Geometry check sheet. Reference: the model listing, model coordinates, mm. A direction names the side the tool comes from. Coordinates: 2 decimals unless noted, no trailing zeros. Loops run counter-clockwise (first coordinate to the right, second up) from the corner with the lowest first, then second, coordinate; pieces in that order, holes last.
from build123d import *

# Parameters (mm, degrees)
SKETCH1_W               = 58
SKETCH1_H               = 48
SKETCH1_R               = 13
SKETCH1_R_2             = 1.8
BOSS_EXTRUDE1_DEPTH     = 5
BOSS_EXTRUDE2_OUTLINE_R = 4.2
BOSS_EXTRUDE2_DEPTH     = 10
FILLET1_R               = 5
BOSS_EXTRUDE5_DEPTH     = 10
CUT_EXTRUDE2_DEPTH      = 67.492480778
SKETCH7_W               = 58
SKETCH7_H               = 5
BOSS_EXTRUDE6_DEPTH     = 13
SKETCH8_R               = 3.3
SKETCH8_R_2             = 1.8
CUT_EXTRUDE3_DEPTH      = 20


# Read off the part's stored shape, not the designer's step: Boss-Extrude2, Boss-Extrude5
with BuildPart() as part:
    # Sketch1 → Boss-Extrude1 (new body)
    with BuildSketch(Plane(origin=(0, 0, 0), x_dir=(1, 0, 0), z_dir=(0, 1, 0))):
        with Locations((29, -24)):
            Rectangle(SKETCH1_W, SKETCH1_H)
        with Locations(Location((35.15, -26.15, 0), (0, 0, 270))):
            Circle(SKETCH1_R, mode=Mode.SUBTRACT)
        with Locations(Location((19.65, -10.65, 0), (0, 0, 270))):
            Circle(SKETCH1_R_2, mode=Mode.SUBTRACT)
        with Locations(Location((19.65, -41.65, 0), (0, 0, 270))):
            Circle(SKETCH1_R_2, mode=Mode.SUBTRACT)
        with Locations(Location((50.65, -41.65, 0), (0, 0, 270))):
            Circle(SKETCH1_R_2, mode=Mode.SUBTRACT)
        with Locations(Location((50.65, -10.65, 0), (0, 0, 270))):
            Circle(SKETCH1_R_2, mode=Mode.SUBTRACT)
    extrude(amount=BOSS_EXTRUDE1_DEPTH)

    # Boss-Extrude2 outline → Boss-Extrude2 (add)
    with BuildSketch(Plane(origin=(0, 5, 0), x_dir=(1, 0, 0), z_dir=(0, 1, 0))):
        with BuildLine():
            ThreePointArc((23.271694215, -31.432598951), (22.15, -26.15), (23.271694215, -20.867401049))
            ThreePointArc((23.271694215, -20.867401049), (8.8, -26.15), (23.271694215, -31.432598951))
        make_face()
        with Locations((17, -26.15)):
            Circle(BOSS_EXTRUDE2_OUTLINE_R, mode=Mode.SUBTRACT)
    extrude(amount=BOSS_EXTRUDE2_DEPTH)

    # Fillet1
    fillet1_edges = [part.edges().sort_by_distance(p)[0] for p in [
        (58, 2.5, 48),
        (0, 2.5, 48),
    ]]
    fillet(fillet1_edges, radius=FILLET1_R)

    # Boss-Extrude5 outline → Boss-Extrude5 (add)
    with BuildSketch(Plane(origin=(0, 5, 0), x_dir=(1, 0, 0), z_dir=(0, 1, 0))):
        with BuildLine():
            ThreePointArc((19.5, -12.443739111), (17.85, -10.65), (19.5, -8.856260889))
            Line((19.5, -8.856260889), (19.5, -5))
            Line((19.5, -5), (14.5, -5))
            Line((14.5, -5), (14.5, -18.340390535))
            ThreePointArc((14.5, -18.340390535), (17, -17.95), (19.5, -18.340390535))
            Line((19.5, -18.340390535), (19.5, -12.443739111))
        make_face()
        with BuildLine():
            ThreePointArc((19.5, -33.959609465), (17, -34.35), (14.5, -33.959609465))
            Line((14.5, -33.959609465), (14.5, -48))
            Line((14.5, -48), (19.5, -48))
            Line((19.5, -48), (19.5, -43.443739111))
            ThreePointArc((19.5, -43.443739111), (17.85, -41.65), (19.5, -39.856260889))
            Line((19.5, -39.856260889), (19.5, -33.959609465))
        make_face()
    extrude(amount=BOSS_EXTRUDE5_DEPTH)

    # Sketch6 → Cut-Extrude2 (cut, through all)
    with BuildSketch(Plane.ZY.offset(-14.5)):
        Polygon((17.340390535, 15), (5, 6), (5, 15), align=None)
        Polygon((48, 6), (34.959609465, 15), (48, 15), align=None)
    extrude(amount=-CUT_EXTRUDE2_DEPTH, mode=Mode.SUBTRACT)

    # Sketch7 → Boss-Extrude6 (add)
    with BuildSketch(Plane(origin=(0, 5, 0), x_dir=(1, 0, 0), z_dir=(0, 1, 0))):
        with Locations((29, -2.5)):
            Rectangle(SKETCH7_W, SKETCH7_H)
    extrude(amount=BOSS_EXTRUDE6_DEPTH)

    # Sketch8 → Cut-Extrude3 (cut)
    with BuildSketch(Plane.XY.offset(5)):
        with Locations((35, 11.5)):
            Circle(SKETCH8_R)
        with Locations((50, 11.5)):
            Circle(SKETCH8_R_2)
    extrude(amount=-CUT_EXTRUDE3_DEPTH, mode=Mode.SUBTRACT)


solid = part.part
(1) Scan lines: L1, parallel to X at y = 2.05, z = 41.65; L2, parallel to Z at x = 35.15, y = 3.8; L3, parallel to Z at x = 19.65, y = 2.1. Record each from-to range of solid material in increasing order.
Findings:
L1: x = 0 to 17.85, 21.45 to 48.85, 52.45 to 58
L2: z = 0 to 13.15, 39.15 to 48
L3: z = 0 to 8.85, 12.45 to 39.85, 43.45 to 48
(2) Sectioned sample at D-D on z = 41. Record the cut outline in (x, y).
Findings:
outline: (0, 0) - (17.97, 0) - (17.97, 10.83) - (14.5, 10.83) - (14.5, 5) - (0, 5) - close; (21.33, 0) - (48.97, 0) - (48.97, 5) - (21.33, 5) - close; (52.33, 0) - (58, 0) - (58, 5) - (52.33, 5) - close
(3) Sectioned sample at A-A on y = 1.75. Record the cut outline in (x, z).
Findings:
outline: (0, 0) - (58, 0) - (58, 43) arc R5 ccw to (53, 48) - (5, 48) arc R5 ccw to (0, 43) - close; hole circle Ø3.6 at (19.65, 10.65); hole circle Ø3.6 at (19.65, 41.65); hole circle Ø26 at (35.15, 26.15); hole circle Ø3.6 at (50.65, 10.65); hole circle Ø3.6 at (50.65, 41.65)
(4) Sectioned sample at B-B on x = 50.65. Record the cut outline in (y, z).
Findings:
outline: (0, 0) - (9.82, 0) - (9.82, 5) - (5, 5) - (5, 8.85) - (0, 8.85) - close; (0, 12.45) - (5, 12.45) - (5, 39.85) - (0, 39.85) - close; (0, 43.45) - (5, 43.45) - (5, 48) - (0, 48) - close; (13.18, 0) - (18, 0) - (18, 5) - (13.18, 5) - close
(5) Draft check along Z on faces 4 (the flat face through (16.96, 10.44, 41.57)), 5 (the cylindrical face through (50.831, 9.903, 2.535)), 6 (the flat face through (14.5, 9, 13)). Enter one of: +Z half, -Z half, draft (parallel to the pull), parting line (faces both ways), or undercut.
Findings:
face 4: +Z half
face 5: draft
face 6: undercut
(6) Gauge pin test, flat ends, axial feed: pin 1 Ø10 at (x, z) = (49, 17) entering from +Y; pin 2 Ø4 at (x, y) = (38, 12.5) entering from +Z; pin 3 Ø16 at (x, z) = (9.5, 30) entering from +Y. Record the tip position at first contact, or that the pin passes through.
Findings:
pin 1: stops at y = 5
pin 2: stops at z = 5
pin 3: stops at y = 15
(7) Sectioned sample at C-C on z = 26.15. Record the cut outline in (x, y), and give its area (4 significant figures).
Findings:
outline: (0, 0) - (22.15, 0) - (22.15, 15) - (21.2, 15) - (21.2, 5) - (12.8, 5) - (12.8, 15) - (8.8, 15) - (8.8, 5) - (0, 5) - close; (48.15, 0) - (58, 0) - (58, 5) - (48.15, 5) - close
area: 209.5 mm2
(8) Access from +Z, -Z, +X, -X, +Y, -Y to the whole of each face (thin tool, end or side, straight path). Record for faces 1 (the flat face through (13, 15, 28)), 2 (the cylindrical face through (21.54, 9.93, 32.98)), 3 (the cylindrical face through (13.67, 9.93, 28.71)).
Findings:
face 1: +Z, +X, -X, +Y
face 2: +Z, +X, +Y
face 3: +Y
